Design review of the part shown in the three views and the two pictorial views. Dimensions are in mm from the part's minimum x, y and z. A direction names the side the tool comes from. Round coordinates to 2 decimals unless told otherwise and drop trailing zeros. Order: outer loops, then holes, each group sorted by start corner. A loop starts at its lowest first (then second) coordinate and runs counter-clockwise, first axis right, second up. Notation, with made-up numbers: M -36.75,-29 L -30.75,-29 A33 ccw -30.75,7 Z; hole C 29,54.25 d1. An arc over 180 degrees is marked long. Write each question's results on one line, items separated by ' | '. Start each with the question number.
Item 1: Machinability: for the marked faces 5, 6 and 7, which of the approach directions +Z, -Z, +X, -X, +Y, -Y give a long, thin tool a straight path to every point of the face, cutting with its end or side? Answer none if there is none.
Item 2: Wall thickness on line 1 (Y direction, x = 29.5, z = 12.7); line 2 (Z direction, x = 23, y = 25); line 3 (X direction, y = 7, z = 14): over which ranges is each line inside the solid? List them lowest first. Write a range as [from, to].
Item 3: Take a section at A-A, the plane y = 25.4. Write out the cut boundary in (x, z), plus the area to 3 significant figures.
Item 4: Take a section at D-D, the plane y = 45. Write out the cut boundary in (x, z).
Item 5: Take a section at B-B, the plane z = 43. Write out the cut boundary in (x, y).
Item 6: Take a section at C-C, the plane x = 39. Write out the cut boundary in (y, z), plus the area to 3 significant figures.
Item 7: Clearance check with flat-ended pins moving along their axes: pin 1 (2 mm diameter, centred on x = 26.5, z = 42.5, fed in from -Y); pin 2 (10 mm diameter, centred on y = 6.5, z = 36.5, fed in from +X); pin 3 (10 mm diameter, centred on x = 56, y = 30, fed in from +Z). State where each tip first meets the part, or that it passes through.
Item 8: The part is to be moulded in two halves that separate along Y. For the marked faces 1, 2, 3 and 4, say which applies: +Y half, -Y half, draft (parallel to the pull), parting line (faces both ways), or undercut.
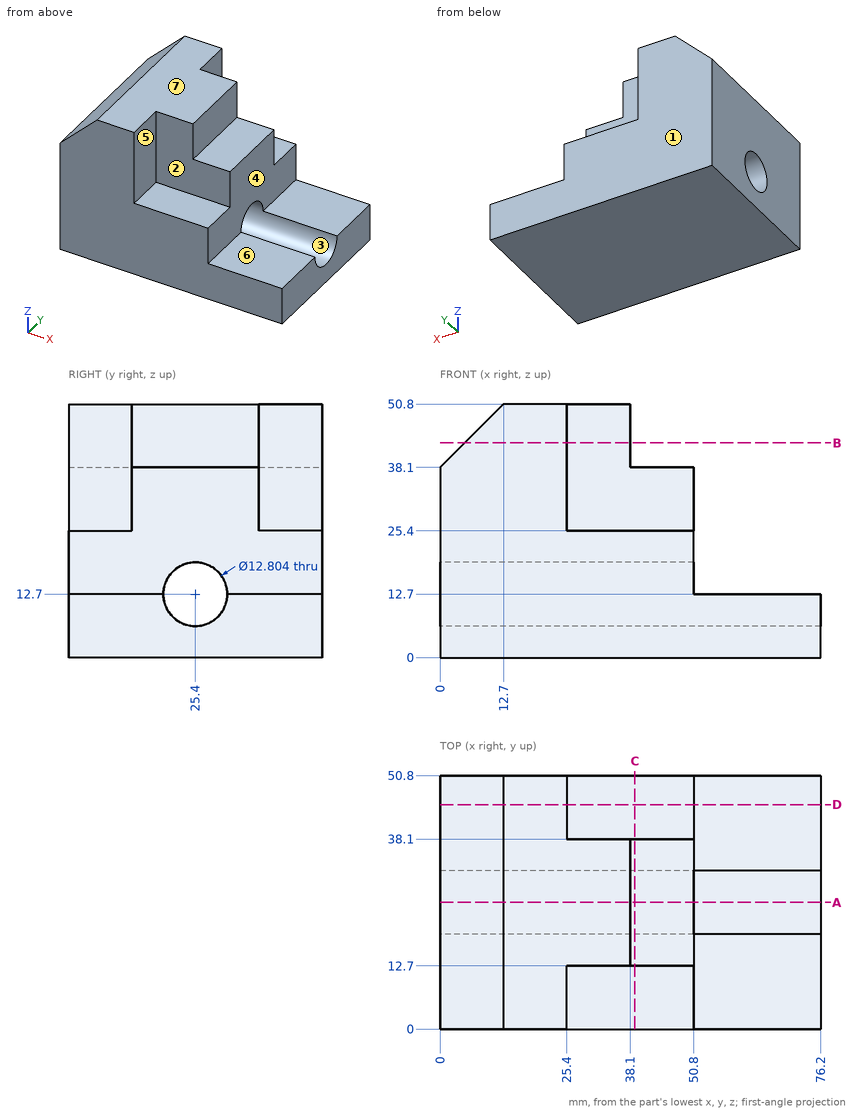
Results list:
1) face 5: +Z, +X, -Y | face 6: +Z, +X, +Y, -Y | face 7: +Z, +X, -X, +Y, -Y
2) line 1: [0, 19], [31.8, 50.8] | line 2: [0, 6.31], [19.09, 50.8] | line 3: [0, 50.8]
3) outline: M 0,0 L 76.2,0 L 76.2,6.3 L 0,6.3 Z; M 0,19.1 L 50.8,19.1 L 50.8,38.1 L 38.1,38.1 L 38.1,50.8 L 12.7,50.8 L 0,38.1 Z | area: 1,850 mm²
4) outline: M 0,0 L 76.2,0 L 76.2,12.7 L 50.8,12.7 L 50.8,25.4 L 25.4,25.4 L 25.4,50.8 L 12.7,50.8 L 0,38.1 Z
5) outline: M 4.9,0 L 25.4,0 L 25.4,12.7 L 38.1,12.7 L 38.1,38.1 L 25.4,38.1 L 25.4,50.8 L 4.9,50.8 Z
6) outline: M 0,0 L 50.8,0 L 50.8,25.4 L 38.1,25.4 L 38.1,38.1 L 12.7,38.1 L 12.7,25.4 L 0,25.4 Z; hole C 25.4,12.7 d12.8 | area: 1,480 mm²
7) pin 1: y = 12.7 | pin 2: x = 25.4 | pin 3: z = 12.7
8) face 1: +Y half | face 2: -Y half | face 3: undercut | face 4: draft
